The listing builds one solid part. Answer for the finished solid, in the listing's coordinates (mm). A direction names the side the tool comes from. Coordinates: 2 decimals unless noted, no trailing zeros. Order: outer loops, then holes, each group sorted by start corner. A loop starts at its lowest first (then second) coordinate and runs counter-clockwise, first axis right, second up. Notation, with made-up numbers: (19.25, 63.25) - (74.25, 63.25) arc R21 cw to (74.25, 79.25) - close; hole circle Ø2 at (76, 57.25). An arc over 180 degrees is marked (long way). Use a Markdown table: item, result. Add a question column.
Item 1: The part is cut by section C-C, the plane z = 4.5. Give the vertices of the cut face in (x, y).
Item 2: The part is cut by section D-D, the plane y = -4.25. Give the vertices of the cut face in (x, z).
Item 3: Find the intervals of material crossed by line 1 along Z through (x, y) = (-24, -1.55); line 2 along X through (y, z) = (-5.5, 15); line 3 along Y through (x, z) = (-16.25, 22), in increasing order.
Item 4: Flat-ended cylindrical pins translate along their axes: P1, Ø1, axis at y = -8.5, z = 23, coming from the -X side; P2, Ø5, axis at x = -18.5, z = 30, coming from the -Y side; P3, Ø1.2, axis at x = -5.5, y = -3.5, coming from the -Z side. Find the tip coordinate at first contact, or state that the pin passes through.
Item 5: The part is cut by section A-A, the plane z = 17. Give the vertices of the cut face in (x, y), then the cut area to 3 significant figures.
Item 6: For faces 1 (the flat face through (-14, 0, 20)), 2 (the flat face through (-7, -5, 11)), 3 (the flat face through (-18, -5, 20)), determine the directions among +Z, -Z, +X, -X, +Y, -Y from which every point of the face is accessible in a straight line to the end or side of a thin tool.
Item 7: The part is cut by section B-B, the plane x = -24. Give the vertices of the cut face in (y, z).
Item 8: The mould has two halves that part along X. Classify faces 4 (the flat face through (-10, -8, 20)), 5 (the cylindrical face through (-25.11, -2.54, 18.01)), 6 (the flat face through (-1, -5, 0)): released by +X, released by -X, zero draft, split by the parting line, or undercut.
Solid Edge part; units mm, degrees
sketch "Sketch1" plane through (0, 0, 0) normal (0, 0, 1) x (1, 0, 0)
  line L0 (-10, -5) -> (-27, -5)
  line L1 (-27, -5) -> (-27, 0)
  line L2 (-27, 0) -> (0, 0)
  line L3 (0, 0) -> (0, -10)
  line L4 (0, -10) -> (-10, -10)
  line L5 (-10, -10) -> (-10, -5)
extrude "Protrusion1" add sketch "Sketch1" along normal blind 40
sketch "Sketch2" plane through (-5, -10, 20) normal (0, -1, 0) x (1, 0, 0)
  line L0 (2, -20) -> (-2, -20)
  line L1 (-2, -20) -> (-2, 3)
  line L2 (-2, 3) -> (2, 3)
  line L3 (2, 3) -> (2, -20)
  dimension "D1" = 2
extrude "VaciadoExtruido_1" cut sketch "Sketch2" against normal blind 50.2328
sketch "Sketch3" plane through (-18.5, -5, 20) normal (0, -1, 0) x (1, 0, 0)
  circle A0 centre (-5.5, 17) radius 1.5
  circle A1 centre (-5.5, -3) radius 1.5
  dimension "D1" = 5.5
extrude "VaciadoExtruido_2" cut sketch "Sketch3" against normal blind 58.7428
Solution:
| question | item | result |
|---|---|---|
| 1 | outline | (-27, -5) - (-10, -5) - (-10, -10) - (-7, -10) - (-7, 0) - (-27, 0) - close; (-3, -10) - (0, -10) - (0, 0) - (-3, 0) - close |
| 2 | outline | (-27, 0) - (-7, 0) - (-7, 23) - (-3, 23) - (-3, 0) - (0, 0) - (0, 40) - (-27, 40) - close; hole circle Ø3 at (-24, 17); hole circle Ø3 at (-24, 37) |
| 3 | line 1 | z = 0 to 15.5, 18.5 to 35.5, 38.5 to 40 |
| 3 | line 2 | x = -10 to -7, -3 to 0 |
| 3 | line 3 | y = -5 to 0 |
| 4 | P1 | stops at x = -10 |
| 4 | P2 | stops at y = -5 |
| 4 | P3 | stops at z = 23 |
| 5 | outline | (-27, -5) - (-25.5, -5) - (-25.5, 0) - (-27, 0) - close; (-22.5, -5) - (-10, -5) - (-10, -10) - (-7, -10) - (-7, 0) - (-22.5, 0) - close; (-3, -10) - (0, -10) - (0, 0) - (-3, 0) - close |
| 5 | area | 130 mm2 |
| 6 | face 1 | +Z, -Z, +X, -X, +Y |
| 6 | face 2 | -Z, +Y, -Y |
| 6 | face 3 | +Z, -Z, -X, -Y |
| 7 | outline | (-5, 0) - (0, 0) - (0, 15.5) - (-5, 15.5) - close; (-5, 18.5) - (0, 18.5) - (0, 35.5) - (-5, 35.5) - close; (-5, 38.5) - (0, 38.5) - (0, 40) - (-5, 40) - close |
| 8 | face 4 | released by -X |
| 8 | face 5 | undercut |
| 8 | face 6 | zero draft |
